Geometry: final body of the model. Coordinates: model frame, mm. A direction names the side the tool comes from. Give positions to 0.01 mm unless a question says otherwise; leave off trailing zeros. Loops run counter-clockwise (first coordinate to the right, second up) from the corner with the lowest first, then second, coordinate; pieces in that order, holes last.
Autodesk Inventor part; units mm, degrees
ref_plane "core_to_washer_XY" through (0, 0, 0) normal (1, 0, 0) x (0, 0, -1)
ref_plane "core_to_washer_YZ" through (0, 0, 0) normal (0, 0, -1) x (0, 1, 0)
ref_plane "core_to_washer_ZX" through (0, 0, 0) normal (0, 1, 0) x (1, 0, 0)
sketch "Sketch_1" plane through (0, 0, 0) normal (0, 0, 1) x (1, 0, 0)
  line L0 (50, 0) -> (-50, 0)
  line L1 (-1, 9.5) -> (-0.75, 9.5)
  line L2 (-0.75, 9.5) -> (-0.75, 8.5)
  line L3 (-0.75, 8.5) -> (0.75, 8.5)
  line L4 (0.75, 8.5) -> (0.75, 9.5)
  line L5 (0.75, 9.5) -> (1, 9.5)
  line L6 (1, 9.5) -> (1, 14.5)
  line L7 (1, 14.5) -> (0.75, 14.5)
  line L8 (0.75, 14.5) -> (0.75, 15)
  line L9 (0.75, 15) -> (-0.75, 15)
  line L10 (-0.75, 15) -> (-0.75, 14.5)
  line L11 (-0.75, 14.5) -> (-1, 14.5)
  line L12 (-1, 14.5) -> (-1, 9.5)
revolve "Revolution1" add sketch "Sketch_1" angle 360 about axis through (50, 0, 0) along (1, 0, 0)
ref_plane "core_to_washer_XY" through (0, 0, 0) normal (1, 0, 0) x (0, 0, -1)
ref_plane "core_to_washer_YZ" through (0, 0, 0) normal (0, 0, -1) x (0, 1, 0)
ref_plane "core_to_washer_ZX" through (0, 0, 0) normal (0, 1, 0) x (1, 0, 0)
ref_plane "core_to_washer1_XY" through (0, 0, 0) normal (-1, 0, 0) x (0, 0, -1)
ref_plane "core_to_washer1_YZ" through (0, 0, 0) normal (0, 0, -1) x (0, -1, 0)
ref_plane "core_to_washer1_ZX" through (0, 0, 0) normal (0, -1, 0) x (-1, 0, 0)
properties part number "core_BA1730"
Item 1: Section query C-C on x = 0.4. Return loops of the section in (y, z).
Values follow:
outline: circle Ø30 at (0, 0); hole circle Ø17 at (0, 0)
Item 2: Section query D-D on z = 12.5. Return loops of the section in (x, y), plus the area to 3 significant figures.
Values follow:
outline: (-1, -7.35) - (-0.75, -7.35) - (-0.75, -8.29) - (0.75, -8.29) - (0.75, -7.35) - (1, -7.35) - (1, 7.35) - (0.75, 7.35) - (0.75, 8.29) - (-0.75, 8.29) - (-0.75, 7.35) - (-1, 7.35) - close
area: 32.2 mm2
Item 3: Set-up query: faces 1 (the face through (0.01, 4.57, 7.167)), 2 (the face through (0.75, -2.2, -8.4)). Return all of +Z, -Z, +X, -X, +Y, -Y with unobstructed straight access to the full face (end or side cutting, diameter ignored); none if empty.
Values follow:
face 1: +X, -X
face 2: +X
Item 4: Section query A-A on y = 0. Return loops of the section in (x, z), plus the area to 3 significant figures.
Values follow:
outline: (-1, -14.5) - (-0.75, -14.5) - (-0.75, -15) - (0.75, -15) - (0.75, -14.5) - (1, -14.5) - (1, -9.5) - (0.75, -9.5) - (0.75, -8.5) - (-0.75, -8.5) - (-0.75, -9.5) - (-1, -9.5) - close; (-1, 9.5) - (-0.75, 9.5) - (-0.75, 8.5) - (0.75, 8.5) - (0.75, 9.5) - (1, 9.5) - (1, 14.5) - (0.75, 14.5) - (0.75, 15) - (-0.75, 15) - (-0.75, 14.5) - (-1, 14.5) - close
area: 24.5 mm2
Item 5: Draft query along Y for faces 3 (the face through (-0.01, -14.985, -0.66)), 4 (the face through (-0.75, -2.2, -8.4)), 5 (the face through (1, 3, -9.5)). Return one class per face: +Y half, -Y half, draft (parallel to the pull), parting line (faces both ways), or undercut.
Values follow:
face 3: parting line
face 4: undercut
face 5: draft
Item 6: Ray query, probe 1 along Z at (x, y) = (0.9, 0); probe 2 along Z at (x, y) = (-0.4, 0); probe 3 along X at (y, z) = (-5.25, -6.75). Return the intervals inside material, ascending.
Values follow:
probe 1: z = -14.5 to -9.5, 9.5 to 14.5
probe 2: z = -15 to -8.5, 8.5 to 15
probe 3: x = -0.75 to 0.75
